Read the model definition and answer for the solid it produces. Units are mm, in the model's axes. A direction names the side the tool comes from. Coordinates: 2 decimals unless noted, no trailing zeros. Write each loop counter-clockwise with the first axis right and the second up, starting at its lowest first coordinate (ties: lowest second). Pieces come first, ordered by that corner, then holes. Notation, with made-up numbers: (21, 54.25) -> (63, 54.25) arc R23 cw to (63, 87.25) -> close; hole circle Ø5 at (-27, -26). An arc over 180 degrees is marked (long way). One line per item, written item: value. Start each with the question number.
1. For faces 4 (the flat face through (0.6, 11, -1.3)), 5 (the flat face through (0.63, 10.01, 1.08)), 6 (the cylindrical face through (1.5, 4.2, -0.07)), determine the directions among +Z, -Z, +X, -X, +Y, -Y from which every point of the face is accessible in a straight line to the end or side of a thin tool.
2. Find section D-D, the plane z = -2.1. Write down the section's boundary in (x, y).
3. Find section C-C, the plane x = -1.85. Write down the section's boundary in (y, z), and give its area (3 significant figures).
4. For a pull along X with two mould halves and no side action, classify faces 1 (the flat face through (0, 0, 0)), 2 (the flat face through (0, 9, 0)), 3 (the cylindrical face through (-0.596, 9.479, -2.685)) as pulls with the +X half, pulls with the -X half, needs draft (parallel to the pull), parting line crosses it, or undercut.
5. Given P1, Ø1, axis at x = 1, y = 9.5, coming from the +Z side; P2, Ø0.8, axis at x = 0, z = 0.5, coming from the +Y side; P3, Ø2, axis at x = -2, y = 9, coming from the -Z side, each flat-ended and moving along its own axis, determine where each tip first touches the part or whether it passes through.
6. Consider line 1 along X through (y, z) = (10, -0.2); line 2 along Z through (x, y) = (0, 4.5); line 3 along Z through (x, y) = (1.2, 4.5). Determine where each line is inside the solid, lowest interval first.
7. Find section B-B, the plane y = 4. Write down the section's boundary in (x, z).
8. Find section A-A, the plane z = 0. Write down the section's boundary in (x, y).
Autodesk Inventor part; units mm, degrees
ref_plane "YZ Plane" through (0, 0, 0) normal (1, 0, 0) x (0, 1, 0)
ref_plane "XZ Plane" through (0, 0, 0) normal (0, 1, 0) x (-1, 0, 0)
ref_plane "XY Plane" through (0, 0, 0) normal (0, 0, 1) x (1, 0, 0)
sketch "Sketch1" plane through (0, 0, 0) normal (0, 1, 0) x (-1, 0, 0)
  circle A0 centre (0, 0) radius 1.5
  dimension "d0" = 3
extrude "Extrusion1" add sketch "Sketch1" along normal blind 8
sketch "Sketch2" plane through (0, 8, 0) normal (0, 1, 0) x (1, 0, 0)
  circle A0 centre (0, 0) radius 1.5
  circle A1 centre (0, 0) radius 2.75
  dimension "d3" = 5.5
extrude "Extrusion2" add sketch "Sketch2" along normal blind 3 contours A0 | A1
sketch "Sketch3" plane through (0, 11, 0) normal (0, 1, 0) x (1, 0, 0)
  circle A0 centre (0, 0) radius 2.75
  line L0 (0, 1.4434) -> (1.25, 0.7217)
  line L1 (1.25, 0.7217) -> (1.25, -0.7217)
  line L2 (1.25, -0.7217) -> (0, -1.4434)
  line L3 (0, -1.4434) -> (-1.25, -0.7217)
  line L4 (-1.25, -0.7217) -> (-1.25, 0.7217)
  line L5 (-1.25, 0.7217) -> (0, 1.4434)
  dimension "d6" = 2.5
extrude "Extrusion3" cut sketch "Sketch3" against normal blind 2 contours L0 L1 L2 L3 L4 L5
thread "Thread1"
chamfer "Chamfer1" distance 0.5 angle 45 1 edges at (1.5, 0, 0)
properties part number "SHCS3x8" material "Stainless Steel"
Answer block:
1. face 4: +Z, -Z, +X, -X, +Y
1. face 5: +Y
1. face 6: -Y
2. outline: (-1.78, 8) -> (1.78, 8) -> (1.78, 11) -> (-1.78, 11) -> close
3. outline: (8, -2.03) -> (11, -2.03) -> (11, 2.03) -> (8, 2.03) -> close
3. area: 12.2 mm2
4. face 1: needs draft
4. face 2: undercut
4. face 3: parting line crosses it
5. P1: stops at z = 2.7
5. P2: stops at y = 9
5. P3: stops at z = -2.56
6. line 1: x = -2.74 to -1.25, 1.25 to 2.74
6. line 2: z = -1.5 to 1.5
6. line 3: z = -0.9 to 0.9
7. outline: circle Ø3 at (0, 0)
8. outline: (-2.75, 8) -> (-1.5, 8) -> (-1.5, 0.5) -> (-1, 0) -> (1, 0) -> (1.5, 0.5) -> (1.5, 8) -> (2.75, 8) -> (2.75, 11) -> (1.25, 11) -> (1.25, 9) -> (-1.25, 9) -> (-1.25, 11) -> (-2.75, 11) -> close
